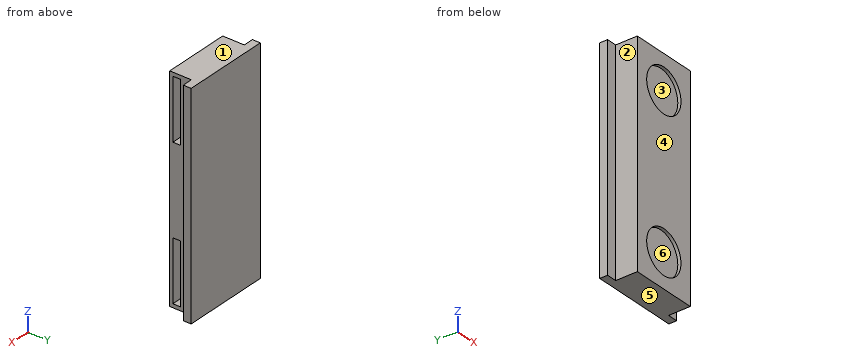
```python
from build123d import *

# Parameters (mm, degrees)
BOSS_EXTRUDE1_DEPTH = 55
SKETCH3_R           = 7.7
CUT_EXTRUDE1_DEPTH  = 2.8
SKETCH4_R           = 7.7
SKETCH4_R_2         = 5.5
BOSS_EXTRUDE2_DEPTH = 0.8
SKETCH5_W           = 15.4
SKETCH5_H           = 2
CUT_EXTRUDE2_DEPTH  = 8.5


with BuildPart() as part:
    # Sketch2 → Boss-Extrude1 (new body)
    with BuildSketch(Plane.XY):
        Polygon((2.6, -2.280794077), (19.6, -2.280794077), (19.6, 3.219205923), (22.2, 3.219205923), (22.2, 5.219205923), (0, 5.219205923), (0, 3.219205923), (2.6, 3.219205923), align=None)
    extrude(amount=-BOSS_EXTRUDE1_DEPTH)

    # Sketch3 → Cut-Extrude1 (cut)
    with BuildSketch(Plane.XZ.offset(2.280794077)):
        with Locations((11.1, -8.64)):
            Circle(SKETCH3_R)
        with Locations((11.1, -46.36)):
            Circle(SKETCH3_R)
    extrude(amount=-CUT_EXTRUDE1_DEPTH, mode=Mode.SUBTRACT)

    # Sketch4 → Boss-Extrude2 (add)
    with BuildSketch(Plane.XZ.offset(2.280794077)):
        with Locations((11.1, -8.64)):
            Circle(SKETCH4_R)
        with Locations((11.1, -8.64)):
            Circle(SKETCH4_R_2, mode=Mode.SUBTRACT)
        with Locations((11.1, -46.36)):
            Circle(SKETCH4_R)
        with Locations((11.1, -46.36)):
            Circle(SKETCH4_R_2, mode=Mode.SUBTRACT)
    extrude(amount=-BOSS_EXTRUDE2_DEPTH)

    # Sketch5 → Cut-Extrude2 (cut)
    with BuildSketch(Plane(origin=(19.6, 0, 0), x_dir=(0, 0, -1), z_dir=(1, 0, 0))):
        with Locations((8.64, -0.480794077)):
            Rectangle(SKETCH5_W, SKETCH5_H)
        with Locations((46.36, -0.480794077)):
            Rectangle(SKETCH5_W, SKETCH5_H)
    extrude(amount=-CUT_EXTRUDE2_DEPTH, mode=Mode.SUBTRACT)


solid = part.part
```
Part model, mm, in its own coordinate system. Face numbers are marked on the shaded views. A direction names the side the tool comes from. Round coordinates to 2 decimals unless told otherwise and drop trailing zeros. Loops run counter-clockwise (first coordinate to the right, second up) from the corner with the lowest first, then second, coordinate; pieces in that order, holes last.
Item 1: Cut at D-D, the plane x = 14. Give the cut face in (y, z), then the cut area to 3 significant figures.
Item 2: Mould opens along Y. For the marked faces 4, 5 and 6 say: +Y half, -Y half, draft (parallel to the pull), parting line (faces both ways), or undercut.
Item 3: Cut at A-A, the plane z = -8.64. Give the cut face in (x, y).
Item 4: Drill centre lines: line 1 (Y direction, x = 10.75, z = -40.5); line 2 (X direction, y = -2, z = -8.64); line 3 (Z direction, x = 18.75, y = -0.5). Where is each one in solid material? Low to high.
Item 5: Cut at B-B, the plane y = -0.5. Give the cut face in (x, z), then the cut area to 3 significant figures.
Item 6: Drop flat-ended pins along their axis: P1, Ø10, axis at x = 11.1, z = -8.64, coming from the -Y side; P2, Ø2, axis at x = 21, z = -32.5, coming from the -Y side; P3, Ø1.6, axis at y = 0, z = -28, coming from the -X side. Give the stop position or say it passes through.
Item 7: 3-axis set-ups, long thin cutter, end or side, ignore diameter. For the marked faces 1, 2 and 3: which of +Z, -Z, +X, -X, +Y, -Y reach the whole face in a straight line?
Item 8: Cut at C-C, the plane z = -30.5. Give the cut face in (x, y), then the cut area to 3 significant figures.
A:
1. outline: (-2.28, -55) - (5.22, -55) - (5.22, 0) - (-2.28, 0) - (-2.28, -3.97) - (-1.48, -3.97) - (-1.48, -0.94) - (0.52, -0.94) - (0.52, -16.34) - (-1.48, -16.34) - (-1.48, -13.31) - (-2.28, -13.31) - (-2.28, -41.69) - (-1.48, -41.69) - (-1.48, -38.66) - (0.52, -38.66) - (0.52, -54.06) - (-1.48, -54.06) - (-1.48, -51.03) - (-2.28, -51.03) - close
1. area: 336 mm2
2. face 4: -Y half
2. face 5: draft
2. face 6: undercut
3. outline: (0, 3.22) - (2.6, 3.22) - (2.6, -2.28) - (5.6, -2.28) - (5.6, -1.48) - (3.4, -1.48) - (3.4, 0.52) - (19.6, 0.52) - (19.6, 3.22) - (22.2, 3.22) - (22.2, 5.22) - (0, 5.22) - close; (16.6, -2.28) - (19.6, -2.28) - (19.6, -1.48) - (16.6, -1.48) - close
4. line 1: y = -2.28 to -1.48, 0.52 to 5.22
4. line 2: x = 2.6 to 5.6, 16.6 to 19.6
4. line 3: z = -55 to -54.06, -38.66 to -16.34, -0.94 to 0
5. outline: (2.6, -55) - (19.6, -55) - (19.6, -54.06) - (11.1, -54.06) arc R7.7 cw to (11.1, -38.66) - (19.6, -38.66) - (19.6, -16.34) - (11.1, -16.34) arc R7.7 cw to (11.1, -0.94) - (19.6, -0.94) - (19.6, 0) - (2.6, 0) - close
5. area: 487 mm2
6. P1: stops at y = 0.52
6. P2: stops at y = 3.22
6. P3: stops at x = 2.6
7. face 1: +Z, +X, -X, +Y, -Y
7. face 2: +Z, -Z, -X, -Y
7. face 3: +X
8. outline: (0, 3.22) - (2.6, 3.22) - (2.6, -2.28) - (19.6, -2.28) - (19.6, 3.22) - (22.2, 3.22) - (22.2, 5.22) - (0, 5.22) - close
8. area: 138 mm2
